```python
from build123d import *

# Parameters (mm, degrees)
SKETCH1_ONE_SIDE_W       = 1.5875
SKETCH1_ONE_SIDE_H       = 18.594090574
BOSS_EXTRUDE1_DEPTH      = 0.3175
BOSS_EXTRUDE1_DEPTH_BACK = 0.3175


with BuildPart() as part:
    # Sketch1 one side → Revolve6 (revolve)
    with BuildSketch(Plane(origin=(0, 0, 0), x_dir=(1, 0, 0), z_dir=(0, 1, 0))):
        with Locations((2.38125, -12.472045287)):
            Rectangle(SKETCH1_ONE_SIDE_W, SKETCH1_ONE_SIDE_H)
    revolve(axis=Axis((0, 0, 0), (0, 0, 1)))

    # Sketch1_10 → Boss-Extrude1 (add, two sides)
    with BuildSketch(Plane(origin=(0, 0, 0), x_dir=(1, 0, 0), z_dir=(0, 1, 0))) as boss_extrude1_sk:
        with BuildLine():
            Line((0, -1.27), (0, -3.175))
            ThreePointArc((0, -3.175), (0.821750468, -3.066814498), (1.5875, -2.749630657))
            Line((1.5875, -2.749630657), (1.5875, 2.749630657))
            Line((1.5875, 2.749630657), (0, 2.749630657))
            Line((0, 2.749630657), (0, 1.27))
            ThreePointArc((0, 1.27), (0.898025612, 0.898025612), (1.27, 0))
            ThreePointArc((1.27, 0), (0.898025612, -0.898025612), (0, -1.27))
        make_face()
        with BuildLine():
            ThreePointArc((-1.5875, -2.749630657), (-0.821750468, -3.066814498), (0, -3.175))
            Line((0, -3.175), (0, -1.27))
            ThreePointArc((0, -1.27), (-1.27, 0), (0, 1.27))
            Line((0, 1.27), (0, 2.749630657))
            Line((0, 2.749630657), (-1.5875, 2.749630657))
            Line((-1.5875, 2.749630657), (-1.5875, -2.749630657))
        make_face()
        with BuildLine():
            ThreePointArc((-3.175, 0), (-2.749630657, -1.5875), (-1.5875, -2.749630657))
            Line((-1.5875, -2.749630657), (-1.5875, 2.749630657))
            ThreePointArc((-1.5875, 2.749630657), (-2.749630657, 1.5875), (-3.175, 0))
        make_face()
        with BuildLine():
            ThreePointArc((0, 3.175), (-0.821750468, 3.066814498), (-1.5875, 2.749630657))
            Line((-1.5875, 2.749630657), (0, 2.749630657))
            Line((0, 2.749630657), (0, 3.175))
        make_face()
        with BuildLine():
            Line((0, 2.749630657), (1.5875, 2.749630657))
            ThreePointArc((1.5875, 2.749630657), (0.821750468, 3.066814498), (0, 3.175))
            Line((0, 3.175), (0, 2.749630657))
        make_face()
        with BuildLine():
            Line((1.5875, 2.749630657), (1.5875, -2.749630657))
            ThreePointArc((1.5875, -2.749630657), (2.749630657, -1.5875), (3.175, 0))
            ThreePointArc((3.175, 0), (2.749630657, 1.5875), (1.5875, 2.749630657))
        make_face()
        with BuildLine():
            Line((-3.175, -3.175), (-1.5875, -3.175))
            Line((-1.5875, -3.175), (-1.5875, -2.749630657))
            ThreePointArc((-1.5875, -2.749630657), (-2.749630657, -1.5875), (-3.175, 0))
            Line((-3.175, 0), (-3.175, -3.175))
        make_face()
        with BuildLine():
            Line((-1.5875, -2.749630657), (-1.5875, -3.175))
            Line((-1.5875, -3.175), (0, -3.175))
            ThreePointArc((0, -3.175), (-0.821750468, -3.066814498), (-1.5875, -2.749630657))
        make_face()
        with BuildLine():
            ThreePointArc((1.5875, -2.749630657), (0.821750468, -3.066814498), (0, -3.175))
            Line((0, -3.175), (1.5875, -3.175))
            Line((1.5875, -3.175), (1.5875, -2.749630657))
        make_face()
        with BuildLine():
            Line((1.5875, -2.749630657), (1.5875, -3.175))
            Line((1.5875, -3.175), (3.175, -3.175))
            Line((3.175, -3.175), (3.175, 0))
            ThreePointArc((3.175, 0), (2.749630657, -1.5875), (1.5875, -2.749630657))
        make_face()
    extrude(amount=BOSS_EXTRUDE1_DEPTH)
    extrude(boss_extrude1_sk.sketch, amount=-BOSS_EXTRUDE1_DEPTH_BACK)


solid = part.part
```
CAD build for the part. Positions are in the model's coordinates, mm. A direction names the side the tool comes from. Round coordinates to 2 decimals unless told otherwise and drop trailing zeros. Order: outer loops, then holes, each group sorted by start corner. A loop starts at its lowest first (then second) coordinate and runs counter-clockwise, first axis right, second up.
Item 1: Saw through at C-C on x = 2.25. Write the cut outline in (y, z) (1 decimal), then the cut area to 3 significant figures.
Item 2: Pin check, flat tips, straight feed: pin 1 (1.9 mm diameter, centred on x = -1.5, z = 0, fed in from +Y); pin 2 (1 mm diameter, centred on y = 2, z = 9, fed in from -X); pin 3 (3 mm diameter, centred on x = -1, y = 2.5, fed in from -Z) (3 decimals). Stop position of each tip, or through.
Item 3: Mould opens along Y. For faces 3 (the face through (0.7, -0.318, 1.4)), 4 (the face through (0, -2, 3.175)), 5 (the face through (-0.207, 1.574, 12.342)) say: pulls with the +Y half, pulls with the -Y half, needs draft (parallel to the pull), parting line crosses it, or undercut.
Item 4: Probe line 1 along X through (y, z) = (0, 16) (1 decimal); line 2 along Z through (x, y) = (2.75, -1) (3 decimals). List the from-to ranges inside material, lowest first.
Item 5: Tool access for faces 1 (the face through (0.7, 0.318, 1.4)), 2 (the face through (-1.4, -1.4, 21.769)): list every direction of +Z, -Z, +X, -X, +Y, -Y with a clear straight run to the whole face (end or side of a thin tool).
Item 6: Saw through at A-A on y = 1. Write the cut outline in (x, z) (3 decimals), then the cut area to 3 significant figures.
Item 7: Saw through at B-B on z = -0.5. Write the cut outline in (x, y).
Reported:
1. outline: (-2.2, 3.2) - (-0.3, 3.2) - (-0.3, -2.2) - (0.3, -2.2) - (0.3, 3.2) - (2.2, 3.2) - (2.2, 21.8) - (-2.2, 21.8) - close
1. area: 86.7 mm2
2. pin 1: stops at y = 0.32
2. pin 2: stops at x = -2.8
2. pin 3: stops at z = 3.175
3. face 3: pulls with the -Y half
3. face 4: needs draft
3. face 5: undercut
4. line 1: x = -3.2 to -1.6, 1.6 to 3.2
4. line 2: z = 3.175 to 21.769
5. face 1: -Z, +X, -X, +Y
5. face 2: +Z, +X, -X, +Y, -Y
6. outline: (-3.013, 3.175) - (-1.233, 3.175) - (-1.233, 21.769) - (-3.013, 21.769) - close; (1.233, 3.175) - (3.013, 3.175) - (3.013, 21.769) - (1.233, 21.769) - close
6. area: 66.2 mm2
7. outline: (-3.14, -0.32) - (-1.17, -0.32) - (-1.17, 0.32) - (-3.14, 0.32) - close; (1.17, -0.32) - (3.14, -0.32) - (3.14, 0.32) - (1.17, 0.32) - close
